from build123d import *

# Parameters (mm, degrees)
BOSS_EXTRUDE1_DEPTH = 10
SKETCH1_3_R         = 5
SKETCH1_3_R_2       = 2
BOSS_EXTRUDE2_DEPTH = 1
BOSS_EXTRUDE3_DEPTH = 20
SKETCH2_R           = 15
BOSS_EXTRUDE4_DEPTH = 2


with BuildPart() as part:
    # Sketch1 → Boss-Extrude1 (new body)
    with BuildSketch(Plane(origin=(0, 0, 0), x_dir=(1, 0, 0), z_dir=(0, 1, 0))):
        with BuildLine():
            Line((2.5, 2.5), (2.5, -2.5))
            ThreePointArc((2.5, -2.5), (0, -5), (-2.5, -2.5))
            Line((-2.5, -2.5), (-2.5, 2.5))
            ThreePointArc((-2.5, 2.5), (0, 5), (2.5, 2.5))
        make_face()
    extrude(amount=-BOSS_EXTRUDE1_DEPTH)

    # Sketch1_3 → Boss-Extrude2 (add)
    with BuildSketch(Plane(origin=(0, 0, 0), x_dir=(1, 0, 0), z_dir=(0, 1, 0))):
        Circle(SKETCH1_3_R)
        with Locations((-0.868240888, -4.924038765)):
            Circle(SKETCH1_3_R_2)
        with Locations((-4.698463104, 1.710100717)):
            Circle(SKETCH1_3_R_2)
        with Locations((4.330127019, 2.5)):
            Circle(SKETCH1_3_R_2)
    extrude(amount=-BOSS_EXTRUDE2_DEPTH)

    # Sketch1_5 → Boss-Extrude3 (add)
    with BuildSketch(Plane(origin=(0, 0, 0), x_dir=(1, 0, 0), z_dir=(0, 1, 0))):
        Polygon((3.742640687, 3.315515147), (4.742640687, 1.583464339), (-3.742640687, -3.315515147), (-4.742640687, -1.583464339), align=None)
    extrude(amount=BOSS_EXTRUDE3_DEPTH)

    # Sketch2 → Boss-Extrude4 (add)
    with BuildSketch(Plane(origin=(-0.500000000000002, 0, -0.8660254037844417), x_dir=(-0.8660254037844386, 0, 0.5000000000000002), z_dir=(-0.5000000000000001, 0, -0.8660254037844385))):
        with Locations((0, 20)):
            Circle(SKETCH2_R)
    extrude(amount=-BOSS_EXTRUDE4_DEPTH)


solid = part.part
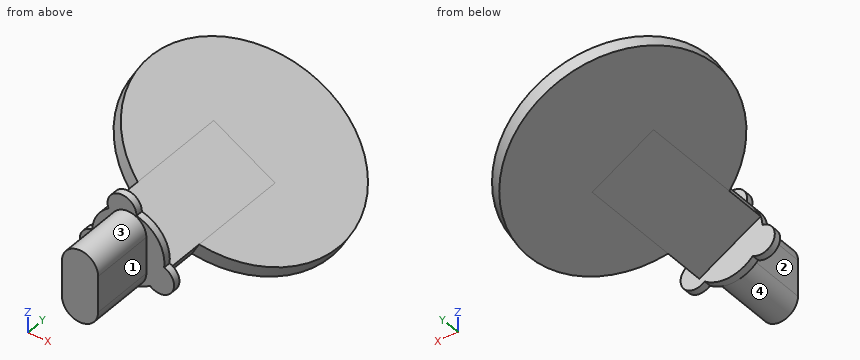
Source: CAD feature listing. Evaluate the final solid. Frame: model axes, mm. Face numbers are marked on the shaded views. A direction names the side the tool comes from. Coordinates: 2 decimals unless noted, no trailing zeros. Loops run counter-clockwise (first coordinate to the right, second up) from the corner with the lowest first, then second, coordinate; pieces in that order, holes last. Notation, with made-up numbers: (-16, 26) -> (-5, 26) arc R37 cw to (-5, 63) -> close; hole circle Ø6 at (30.25, 79). An arc over 180 degrees is marked (long way). Answer in a Markdown table with one row per item. Add a question column.
Q1. Section B-B on y = 8. Return the cut outline in (x, z).
Q2. Ray query, line 1 along X through (y, z) = (9, 0.5); line 2 along Y through (x, z) = (-2.25, 5.75); line 3 along Z through (x, y) = (1.5, 16). Return the intervals inside material, ascending.
Q3. Section A-A on y = 16.5. Return the cut outline in (x, z), and give its area (3 significant figures).
Q4. Reachability of the marked faces 1, 2, 3 and 4 from +Z, -Z, +X, -X, +Y, -Y: full face, straight path, thin tool, end or side. Return the list, or none.
Q5. Section D-D on y = 26.5. Return the cut outline in (x, z), and give its area (3 significant figures).
Q6. Contact query for flat-ended pins moving along their axis: pin 1 Ø5.5 at (y, z) = (-5.5, -0.5) entering from -X; pin 2 Ø1.5 at (x, y) = (-5.5, 9) entering from -Z; pin 3 Ø6 at (y, z) = (8, 5) entering from +X. Output: stop coordinate, or through.
Q7. Section C-C on y = 3.5. Return the cut outline in (x, z), and give its area (3 significant figures).
Computed values:
| question | item | result |
|---|---|---|
| 1 | outline | (-8.29, 3.63) -> (7.29, -5.37) -> (8.29, -3.63) -> (-7.29, 5.37) -> close |
| 2 | line 1 | x = -2.87 to 1.13 |
| 2 | line 2 | y = -1 to 0 |
| 2 | line 3 | z = -2.02 to 0.29 |
| 3 | outline | (-13.13, 6.43) -> (12.13, -8.16) -> (13.13, -6.43) -> (-12.13, 8.16) -> close |
| 3 | area | 58.3 mm^2 |
| 4 | face 1 | +Z, -Z, +X, -Y |
| 4 | face 2 | +Z, -Z, -X, -Y |
| 4 | face 3 | +Z, -Y |
| 4 | face 4 | -Z, -Y |
| 5 | outline | (-12.21, 5.89) -> (11.21, -7.63) -> (12.21, -5.89) -> (-11.21, 7.63) -> close |
| 5 | area | 54.1 mm^2 |
| 6 | pin 1 | stops at x = -2.5 |
| 6 | pin 2 | stops at z = 1.59 |
| 6 | pin 3 | stops at x = -1.46 |
| 7 | outline | (-4.74, 1.58) -> (3.74, -3.32) -> (4.74, -1.58) -> (-3.74, 3.32) -> close |
| 7 | area | 19.6 mm^2 |
